from build123d import *

# Parameters (mm, degrees)
F0_R     = 0.75
F1_DEPTH = 1
F3_DEPTH = 1.0010001
F2_R     = 0.9
F2_R_2   = 0.75
F4_DEPTH = 1.0010001


with BuildPart() as f1:
    # F0 (on Top) → F1 (new body)
    with BuildSketch(Plane.XY):
        with BuildLine():
            Line((8.4099927317, 7.5580001656), (5.0252605515, 20.6268022556))
            ThreePointArc((5.0252605515, 20.6268022556), (1.9783097607, 22.4201485352), (0.1849634811, 19.3731977444))
            Line((0.1849634811, 19.3731977444), (0.9371261878, 16.4690195022))
            ThreePointArc((0.9371261878, 16.4690195022), (0.8653051518, 15.2434273388), (0.0910006691, 14.2907012605))
            ThreePointArc((0.0910006691, 14.2907012605), (0.024216232, 14.2184078876), (0, 14.1230136168))
            Line((0, 14.1230136168), (0, 3.5349456812))
            add(Edge.make_bspline(
                [(0, 3.5349456812), (0, 0.1151861329), (2.5847140193, 0.0126293901)],
                knots=[4.7123889804, 4.7123889804, 4.7123889804, 6.2531913499, 6.2531913499, 6.2531913499], degree=2, weights=[1, 0.717631333, 1]))
            ThreePointArc((2.5847140193, 0.0126293901), (8.1188853822, 0.7647703189), (13.0609901745, 3.3663792197))
            ThreePointArc((13.0609901745, 3.3663792197), (13.3106896342, 3.672880965), (13.4, 4.0580001656))
            Line((13.4, 4.0580001656), (13.4, 7.0580001656))
            ThreePointArc((13.4, 7.0580001656), (13.2535533906, 7.4115535562), (12.9, 7.5580001656))
            Line((12.9, 7.5580001656), (8.4099927317, 7.5580001656))
        make_face()
        with BuildLine():
            ThreePointArc((3.1154618928, 6.4541634531), (5.0869565217, 9.8093739335), (4.8362002383, 5.9259025835))
            Line((4.8362002383, 5.9259025835), (4.0103691728, 3.2358695652))
            ThreePointArc((4.0103691728, 3.2358695652), (2.8858695652, 2.6396308272), (2.2896308272, 3.7641304348))
            Line((2.2896308272, 3.7641304348), (3.1154618928, 6.4541634531))
        make_face(mode=Mode.SUBTRACT)
        with Locations((2.6051120163, 20)):
            Circle(F0_R, mode=Mode.SUBTRACT)
    extrude(amount=F1_DEPTH)

    # F2 (on face) → F3 (cut, through all)
    with BuildSketch(Plane.XY.offset(1)):
        with BuildLine():
            Line((3.1154618928, 6.4541634531), (3.0504773302, 6.2424850283))
            ThreePointArc((3.0504773302, 6.2424850283), (3.8543478261, 5.794317794), (4.7712156757, 5.7142241587))
            Line((4.7712156757, 5.7142241587), (4.8362002383, 5.9259025835))
            ThreePointArc((4.8362002383, 5.9259025835), (4.8920816578, 5.9362509706), (4.9476464888, 5.9481829327))
            Line((4.9476464888, 5.9481829327), (5.4559657475, 7.6039641776))
            ThreePointArc((5.4559657475, 7.6039641776), (4.2065217391, 6.941476691), (3.5440342525, 8.1909206994))
            Line((3.5440342525, 8.1909206994), (3.0357149938, 6.5351394544))
            ThreePointArc((3.0357149938, 6.5351394544), (3.0750131365, 6.4940848793), (3.1154618928, 6.4541634531))
        make_face()
        with BuildLine():
            ThreePointArc((4.8808681557, 5.7306615433), (6.1849198709, 6.4828594509), (6.7, 7.8974424385))
            ThreePointArc((6.7, 7.8974424385), (3.6421944703, 9.9233174774), (2.9689366607, 6.317618065))
            Line((2.9689366607, 6.317618065), (3.0357149938, 6.5351394544))
            ThreePointArc((3.0357149938, 6.5351394544), (5.0869565217, 9.8093739335), (4.9476464888, 5.9481829327))
            Line((4.9476464888, 5.9481829327), (4.8808681557, 5.7306615433))
        make_face()
        with BuildLine():
            ThreePointArc((4.7712156757, 5.7142241587), (4.8261454855, 5.7217519453), (4.8808681557, 5.7306615433))
            Line((4.8808681557, 5.7306615433), (4.9476464888, 5.9481829327))
            ThreePointArc((4.9476464888, 5.9481829327), (4.8920816578, 5.9362509706), (4.8362002383, 5.9259025835))
            Line((4.8362002383, 5.9259025835), (4.7712156757, 5.7142241587))
        make_face()
        with BuildLine():
            Line((3.0357149938, 6.5351394544), (2.9689366607, 6.317618065))
            ThreePointArc((2.9689366607, 6.317618065), (3.0092335922, 6.2795377697), (3.0504773302, 6.2424850283))
            Line((3.0504773302, 6.2424850283), (3.1154618928, 6.4541634531))
            ThreePointArc((3.1154618928, 6.4541634531), (3.0750131365, 6.4940848793), (3.0357149938, 6.5351394544))
        make_face()
        with BuildLine():
            ThreePointArc((4.9476464888, 5.9481829327), (5.0869565217, 9.8093739335), (3.0357149938, 6.5351394544))
            Line((3.0357149938, 6.5351394544), (3.5440342525, 8.1909206994))
            ThreePointArc((3.5440342525, 8.1909206994), (4.6483816911, 8.8863726048), (5.5, 7.8974424385))
            ThreePointArc((5.5, 7.8974424385), (5.4889301663, 7.7490607474), (5.4559657475, 7.6039641776))
            Line((5.4559657475, 7.6039641776), (4.9476464888, 5.9481829327))
        make_face()
    extrude(amount=-F3_DEPTH, mode=Mode.SUBTRACT)

    # F2 (on face) → F4 (cut, through all)
    with BuildSketch(Plane.XY.offset(1)):
        with Locations((2.6051120163, 20)):
            Circle(F2_R)
        with Locations((2.6051120163, 20)):
            Circle(F2_R_2, mode=Mode.SUBTRACT)
    extrude(amount=-F4_DEPTH, mode=Mode.SUBTRACT)


solid = f1.part
Here's how the part is built. I have some questions about the finished solid (model axes, mm). A direction names the side the tool comes from. Round coordinates to 2 decimals unless told otherwise and drop trailing zeros. Write each loop counter-clockwise with the first axis right and the second up, starting at its lowest first coordinate (ties: lowest second). Pieces come first, ordered by that corner, then holes.
1. Will this pin go through, and if not, where does the flat tip stop? pin 1 Ø1.4 at (x, y) = (2.61, 20) entering from +Z.
2. For faces 1 (the flat face through (2.665, 4.986, 0.493)), 2 (the flat face through (10.7, 7.558, 0.5)), 3 (the flat face through (13.4, 5.5, 0.5)), which set-ups out of +Z, -Z, +X, -X, +Y, -Y let a thin tool reach every point of the face, with its end or its side?
3. Suppose I cut it at C-C (z = 0.8). State how many separate pieces and enclosed holes the cut face has, and give its area (3 significant figures).
4. If we mould it in two halves opening along Y, with no side actions, what happens to faces 4 (the flat face through (7, 9, 1)), 5 (the flat face through (0.556, 17.941, 0.493)), 6 (the flat face through (4.4, 4.5, 0.5)), 7 (the cylindrical face through (8.04, 0.74, 0.49))? For each: released by +Y, released by -Y, zero draft, split by the parting line, or undercut.
5. Suppose I cut it at A-A (x = 4.5). List the corners of the cut face in (y, z) for me.
6. Suppose I cut it at B-B (y = 20.25). List the corners of the cut face in (x, z) for me, and give its area (3 significant figures).
7. I need wall thicknesses on L1, parallel to X at y = 19.25, z = 0.1; L2, parallel to X at y = 8, z = 0.9; L3, parallel to Y at x = 3.75, z = 0.1. Which ranges of each line are inside material? Lowest first, please.
8. Suppose I cut it at D-D (x = 8). List the corners of the cut face in (y, z) for me, and give its area (3 significant figures).
Answer sheet:
1. pin 1: passes through
2. face 1: +Z, -Z
2. face 2: +Z, -Z, +X, +Y
2. face 3: +Z, -Z, +X, +Y, -Y
3. separate pieces: 1
3. enclosed holes: 2
3. area: 155 mm2
4. face 4: zero draft
4. face 5: undercut
4. face 6: undercut
4. face 7: released by -Y
5. outline: (0.05, 0) - (4.83, 0) - (4.83, 1) - (0.05, 1) - close; (10.1, 0) - (21.63, 0) - (21.63, 1) - (10.1, 1) - close
6. outline: (0.12, 0) - (1.74, 0) - (1.74, 1) - (0.12, 1) - close; (3.47, 0) - (5.12, 0) - (5.12, 1) - (3.47, 1) - close
6. area: 3.28 mm2
7. L1: x = 0.22 to 2.11, 3.1 to 5.38
7. L2: x = 0 to 2.3, 6.7 to 8.3
7. L3: y = 0.01 to 2.83, 9.97 to 22.22
8. outline: (0.73, 0) - (9.14, 0) - (9.14, 1) - (0.73, 1) - close
8. area: 8.41 mm2
